```python
from build123d import *

# Parameters (mm, degrees)
F0_W      = 280
F0_H      = 120
F1_DEPTH  = 20
F2_W      = 160
F2_H      = 120
F3_DEPTH  = 10
F5_DEPTH  = 25
F6_W      = 40
F6_H      = 120
F7_DEPTH  = 10
F9_DEPTH  = 10.001
F11_DEPTH = 240.001
F12_SIZE  = 0.5
F13_SIZE  = 0.5
F14_SIZE  = 0.5


with BuildPart() as f1:
    # F0 (on Front) → F1 (new body)
    with BuildSketch(Plane.XZ):
        Rectangle(F0_W, F0_H)
    extrude(amount=F1_DEPTH)

    # F2 (on face) → F3 (cut)
    with BuildSketch(Plane.XZ.offset(20)):
        with Locations((-60, 0)):
            Rectangle(F2_W, F2_H)
    extrude(amount=-F3_DEPTH, mode=Mode.SUBTRACT)

    # F4 (on face) → F5 (cut)
    with BuildSketch(Plane.XZ.offset(10)):
        with BuildLine():
            Line((-105, -20), (-55, -20))
            ThreePointArc((-55, -20), (-51.4644660941, -18.5355339059), (-50, -15))
            Line((-50, -15), (-50, 15))
            ThreePointArc((-50, 15), (-51.4644660941, 18.5355339059), (-55, 20))
            Line((-55, 20), (-105, 20))
            ThreePointArc((-105, 20), (-108.5355339059, 18.5355339059), (-110, 15))
            Line((-110, 15), (-110, -15))
            ThreePointArc((-110, -15), (-108.5355339059, -18.5355339059), (-105, -20))
        make_face()
    extrude(amount=-F5_DEPTH, mode=Mode.SUBTRACT)

    # F6 (on face) → F7 (cut)
    with BuildSketch(Plane.XZ.offset(20)):
        with Locations((120, 0)):
            Rectangle(F6_W, F6_H)
    extrude(amount=-F7_DEPTH, mode=Mode.SUBTRACT)

    # F8 (on face) → F9 (cut, through all)
    with BuildSketch(Plane.XZ.offset(10)):
        with BuildLine():
            ThreePointArc((110, -25), (111.4644660941, -28.5355339059), (115, -30))
            Line((115, -30), (125, -30))
            ThreePointArc((125, -30), (128.5355339059, -28.5355339059), (130, -25))
            Line((130, -25), (130, 25))
            ThreePointArc((130, 25), (128.5355339059, 28.5355339059), (125, 30))
            Line((125, 30), (115, 30))
            ThreePointArc((115, 30), (111.4644660941, 28.5355339059), (110, 25))
            Line((110, 25), (110, -25))
        make_face()
    extrude(amount=-F9_DEPTH, mode=Mode.SUBTRACT)

    # F10 (on face) → F11 (cut, through all)
    with BuildSketch(Plane.YZ.offset(100)):
        Polygon((-18.25, -51.25), (-17, -51.25), (-17, -48.75), (-18.25, -48.75), (-20, -47), (-20, -53), align=None)
        Polygon((-20, -37), (-20, -43), (-18.25, -41.25), (-17, -41.25), (-17, -38.75), (-18.25, -38.75), align=None)
        Polygon((-20, -27), (-20, -33), (-18.25, -31.25), (-17, -31.25), (-17, -28.75), (-18.25, -28.75), align=None)
        Polygon((-20, -17), (-20, -23), (-18.25, -21.25), (-17, -21.25), (-17, -18.75), (-18.25, -18.75), align=None)
        Polygon((-20, -7), (-20, -13), (-18.25, -11.25), (-17, -11.25), (-17, -8.75), (-18.25, -8.75), align=None)
        Polygon((-20, 3), (-20, -3), (-18.25, -1.25), (-17, -1.25), (-17, 1.25), (-18.25, 1.25), align=None)
        Polygon((-20, 13), (-20, 7), (-18.25, 8.75), (-17, 8.75), (-17, 11.25), (-18.25, 11.25), align=None)
        Polygon((-20, 23), (-20, 17), (-18.25, 18.75), (-17, 18.75), (-17, 21.25), (-18.25, 21.25), align=None)
        Polygon((-20, 33), (-20, 27), (-18.25, 28.75), (-17, 28.75), (-17, 31.25), (-18.25, 31.25), align=None)
        Polygon((-20, 43), (-20, 37), (-18.25, 38.75), (-17, 38.75), (-17, 41.25), (-18.25, 41.25), align=None)
        Polygon((-20, 53), (-20, 47), (-18.25, 48.75), (-17, 48.75), (-17, 51.25), (-18.25, 51.25), align=None)
    extrude(amount=-F11_DEPTH, mode=Mode.SUBTRACT)

    # F12
    f12_edges = [f1.edges().sort_by_distance(p)[0] for p in [
        (60, -20, -60),
        (100, -20, -56.5),
        (100, -20, -45),
        (100, -20, -25),
        (100, -20, -15),
        (100, -20, -35),
        (100, -20, -5),
        (100, -20, 5),
        (100, -20, 15),
        (100, -20, 25),
        (100, -20, 35),
        (100, -20, 45),
        (100, -20, 56.5),
        (60, -20, 60),
        (20, -20, -56.5),
        (20, -20, -45),
        (20, -20, -35),
        (20, -20, -25),
        (20, -20, -15),
        (20, -20, -5),
        (20, -20, 5),
        (20, -20, 15),
        (20, -20, 25),
        (20, -20, 56.5),
        (20, -20, 45),
        (20, -20, 35),
    ]]
    chamfer(f12_edges, length=F12_SIZE)

    # F13
    f13_edges = [f1.edges().sort_by_distance(p)[0] for p in [
        (110, -10, 0),
        (-80, -10, -20),
        (-80, 0, -20),
        (110, 0, 0),
    ]]
    chamfer(f13_edges, length=F13_SIZE)

    # F14
    f14_edges = [f1.edges().sort_by_distance(p)[0] for p in [
        (-140, -5, 60),
        (-140, -10, 0),
        (-140, 0, 0),
        (-140, -5, -60),
        (-60, -10, 60),
        (0, 0, 60),
        (20, -14.75, 60),
        (20, -14.75, -60),
        (-60, -10, -60),
        (0, 0, -60),
        (140, -5, 60),
        (140, 0, 0),
        (140, -10, 0),
        (140, -5, -60),
        (100, -14.75, 60),
        (120, -10, 60),
        (120, -10, -60),
        (100, -14.75, -60),
    ]]
    chamfer(f14_edges, length=F14_SIZE)


solid = f1.part
```
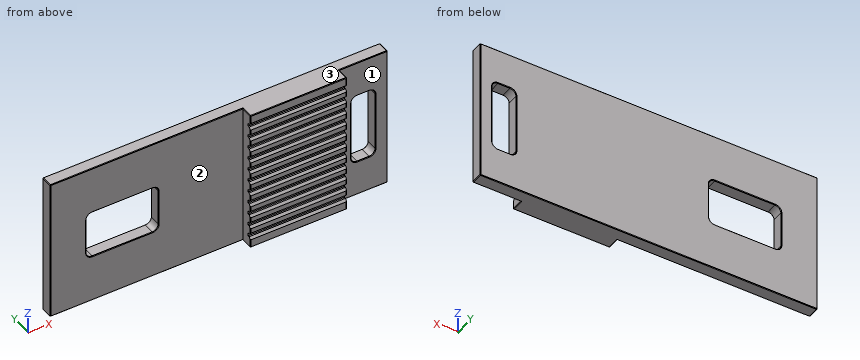
Design review of the part built by this model. Coordinates are the model's own, in mm. Face numbers are marked on the shaded views. A direction names the side the tool comes from. Coordinates: 2 decimals unless noted, no trailing zeros. Loops run counter-clockwise (first coordinate to the right, second up) from the corner with the lowest first, then second, coordinate; pieces in that order, holes last.
Q1. Tool access review of the marked faces 1, 2 and 3: name each direction out of +Z, -Z, +X, -X, +Y, -Y from which nothing blocks a thin tool from reaching the whole face with its end or side.
Reported:
face 1: +Z, -Z, +X, -Y
face 2: +Z, -Z, -X, -Y
face 3: +Z, +X, -X, +Y, -Y
Q2. For pin 1 (2 mm diameter, centred on x = 66.5, z = 20, fed in from -Y); pin 2 (3 mm diameter, centred on x = 79.5, z = 10.5, fed in from -Y); pin 3 (3 mm diameter, centred on y = -17, z = 20.5, fed in from +X), all flat-tipped, find the tip position at first contact; note any pin that passes through.
Reported:
pin 1: stops at y = -17
pin 2: stops at y = -19
pin 3: stops at x = 100
Q3. We need section A-A on y = -4. State the section outline as (x, z) points, and give its area (3 significant figures).
Reported:
outline: (-140, -59.5) - (-139.5, -60) - (139.5, -60) - (140, -59.5) - (140, 59.5) - (139.5, 60) - (-139.5, 60) - (-140, 59.5) - close; hole (-110, -15) arc R5 ccw to (-105, -20) - (-55, -20) arc R5 ccw to (-50, -15) - (-50, 15) arc R5 ccw to (-55, 20) - (-105, 20) arc R5 ccw to (-110, 15) - close; hole (110, -25) arc R5 ccw to (115, -30) - (125, -30) arc R5 ccw to (130, -25) - (130, 25) arc R5 ccw to (125, 30) - (115, 30) arc R5 ccw to (110, 25) - close
area: 30,000 mm2
Q4. We need section B-B on x = -16.5. State the section outline as (y, z) points.
Reported:
outline: (-10, -59.5) - (-9.5, -60) - (-0.5, -60) - (0, -59.5) - (0, 59.5) - (-0.5, 60) - (-9.5, 60) - (-10, 59.5) - close
Q5. To check wall thickness, follow line 1 (X direction, y = -2, z = 4.5); line 2 (Z direction, x = -105.5, y = -2.5); line 3 (Y direction, x = -31.5, z = 14.5). State the ranges of each line that lie inside material, in increasing order.
Reported:
line 1: x = -140 to -110, -50 to 110, 130 to 140
line 2: z = -60 to -19.97, 19.97 to 60
line 3: y = -10 to 0
